Geometry check sheet. Reference: the model listing, model coordinates, mm. A direction names the side the tool comes from. Give positions to 0.01 mm unless a question says otherwise; leave off trailing zeros. Order: outer loops, then holes, each group sorted by start corner. A loop starts at its lowest first (then second) coordinate and runs counter-clockwise, first axis right, second up. Notation, with made-up numbers: M 44,-22 L 95,-22 A29 cw 95,16 Z; hole C -35,54.5 d8. An arc over 180 degrees is marked long. Put each result on its own line as item: value. Start each with the question number.
Q1. Access from +Z, -Z, +X, -X, +Y, -Y to the whole of each face (thin tool, end or side, straight path). Record for faces 1 (the flat face through (5.5, 1, 1)), 2 (the cylindrical face through (-6, 1, 0)), 3 (the flat face through (-7.5, 2, 0)).
Q2. Section check D-D on y = 0.4. Record the cut outline in (x, z), then the cut area to 3 significant figures.
Q3. Material ranges on L1, parallel to X at y = 0.25, z = 1.75; L2, parallel to Y at x = 6.25, z = 0.4; L3, parallel to Y at x = -6, z = 0.2, recorded low to high.
Q4. Section check C-C on z = 1.35. Record the cut outline in (x, y).
Q5. Section check A-A on z = 0. Record the cut outline in (x, y), then the cut area to 3 significant figures.
Q6. Section check B-B on y = 2. Record the cut outline in (x, z).
```python
from build123d import *

# Parameters (mm, degrees)
SKETCH1_W           = 11
SKETCH1_H           = 4
BOSS_EXTRUDE1_DEPTH = 4
SKETCH2_R           = 1
BOSS_EXTRUDE2_DEPTH = 2
SKETCH3_R           = 1
BOSS_EXTRUDE3_DEPTH = 2


with BuildPart() as part:
    # Sketch1 → Boss-Extrude1 (new body)
    with BuildSketch(Plane(origin=(0, 0, 0), x_dir=(1, 0, 0), z_dir=(0, 1, 0))):
        Rectangle(SKETCH1_W, SKETCH1_H)
    extrude(amount=BOSS_EXTRUDE1_DEPTH)

    # Sketch2 → Boss-Extrude2 (add)
    with BuildSketch(Plane(origin=(5.5, 0, 0), x_dir=(0, 0, -1), z_dir=(1, 0, 0))):
        with Locations((0, 2)):
            Circle(SKETCH2_R)
    extrude(amount=BOSS_EXTRUDE2_DEPTH)

    # Sketch3 → Boss-Extrude3 (add)
    with BuildSketch(Plane.ZY.offset(5.5)):
        with Locations((0, 2)):
            Circle(SKETCH3_R)
    extrude(amount=BOSS_EXTRUDE3_DEPTH)


solid = part.part
```
Results found:
1. face 1: +X
1. face 2: -X
1. face 3: +Z, -Z, -X, +Y, -Y
2. outline: M -5.5,-2 L 5.5,-2 L 5.5,2 L -5.5,2 Z
2. area: 44.0 mm^2
3. L1: x = -5.5 to 5.5
3. L2: y = 1.08 to 2.92
3. L3: y = 1.02 to 2.98
4. outline: M -5.5,0 L 5.5,0 L 5.5,4 L -5.5,4 Z
5. outline: M -7.5,1 L -5.5,1 L -5.5,0 L 5.5,0 L 5.5,1 L 7.5,1 L 7.5,3 L 5.5,3 L 5.5,4 L -5.5,4 L -5.5,3 L -7.5,3 Z
5. area: 52.0 mm^2
6. outline: M -7.5,-1 L -5.5,-1 L -5.5,-2 L 5.5,-2 L 5.5,-1 L 7.5,-1 L 7.5,1 L 5.5,1 L 5.5,2 L -5.5,2 L -5.5,1 L -7.5,1 Z
